Geometry check sheet. Reference: the model listing, model coordinates, mm. Give positions to 0.01 mm unless a question says otherwise; leave off trailing zeros. Write each loop counter-clockwise with the first axis right and the second up, starting at its lowest first coordinate (ties: lowest second). Pieces come first, ordered by that corner, then holes. Notation, with made-up numbers: (57, 38.5) -> (69, 38.5) arc R19 cw to (69, 59.5) -> close; hole circle Ø3 at (32, -5). An arc over 180 degrees is marked (long way). Write item = value, one per line. Start each with the question number.
1. Mould release check, pull along Z, two halves, no side actions. Record for faces 1 (the flat face through (-1, 5, -2)), 2 (the cylindrical face through (3, 3, 0)), 3 (the flat face through (0.961, 2.535, -1.695)): pulls with the +Z half, pulls with the -Z half, needs draft (parallel to the pull), parting line crosses it, or undercut.
2. Thickness scan on line 1 along X through (y, z) = (1.45, -0.75); line 2 along Z through (x, y) = (1.75, 0.65); line 3 along X through (y, z) = (4.85, 2). Record the ranges inside material, lowest first.
3. Cross-section at A-A, the plane z = 0. Record the cut outline in (x, y).
4. Cross-section at C-C, the plane y = 0.6. Record the cut outline in (x, z) (3 decimals).
5. Cross-section at B-B, the plane y = 3.15. Record the cut outline in (x, z) (3 decimals), plus the area to 3 significant figures.
6. Depth check by flat-ended pin: P1, Ø2, axis at x = -2, y = 4, coming from the -Z side; P2, Ø1.5, axis at y = 2, z = -1.5, coming from the -X side. Enter the tip coordinate at first touch or a pass-through.
Autodesk Inventor part; units mm, degrees
ref_plane "YZ Plane" through (0, 0, 0) normal (1, 0, 0) x (0, 1, 0)
ref_plane "XZ Plane" through (0, 0, 0) normal (0, 1, 0) x (-1, 0, 0)
ref_plane "XY Plane" through (0, 0, 0) normal (0, 0, 1) x (1, 0, 0)
sketch "Sketch1" plane through (0, 0, 0) normal (0, 1, 0) x (-1, 0, 0)
  circle A0 centre (0, 0) radius 2.25
  circle A1 centre (0, 0) radius 3
  dimension "d0" = 4.5
  dimension "d1" = 6
extrude "Extrusion1" add sketch "Sketch1" along normal blind 5 contours A0 | A1
sketch "Sketch2" plane through (0, 5, 0) normal (0, 1, 0) x (1, 0, 0)
  line L0 (0, 0) -> (0, 2.25)
  line L1 (0, 2.25) -> (1.9486, 1.125)
  line L2 (1.9486, 1.125) -> (1.9486, -1.125)
  line L3 (1.9486, -1.125) -> (0, -2.25)
  line L4 (0, -2.25) -> (-1.9486, -1.125)
  line L5 (-1.9486, -1.125) -> (-1.9486, 1.125)
  line L6 (-1.9486, 1.125) -> (0, 2.25)
  dimension "d4" = 2.25
extrude "Extrusion2" cut sketch "Sketch2" against normal through all
fillet "Fillet2" radius 1 1 edges at (3, 0, 0)
properties part number "Nut"
Answers:
q1.face_1 = needs draft
q1.face_2 = parting line crosses it
q1.face_3 = undercut
q2.line_1 = -2.9 to -1.95, 1.95 to 2.9
q2.line_2 = -2.36 to -1.24, 1.24 to 2.36
q2.line_3 = -2.24 to -0.43, 0.43 to 2.24
q3.outline = (-3, 1) arc R1 ccw to (-2, 0) -> (-1.95, 0) -> (-1.95, 5) -> (-3, 5) -> close; (1.95, 0) -> (2, 0) arc R1 ccw to (3, 1) -> (3, 5) -> (1.95, 5) -> close
q4.outline = circle Ø5.833 at (0, 0); hole (-1.949, -1.125) -> (0, -2.25) -> (1.949, -1.125) -> (1.949, 1.125) -> (0, 2.25) -> (-1.949, 1.125) -> close
q5.outline = circle Ø6 at (0, 0); hole (-1.949, -1.125) -> (0, -2.25) -> (1.949, -1.125) -> (1.949, 1.125) -> (0, 2.25) -> (-1.949, 1.125) -> close
q5.area = 15.1 mm^2
q6.P1 = -2.83
q6.P2 = -2.9
